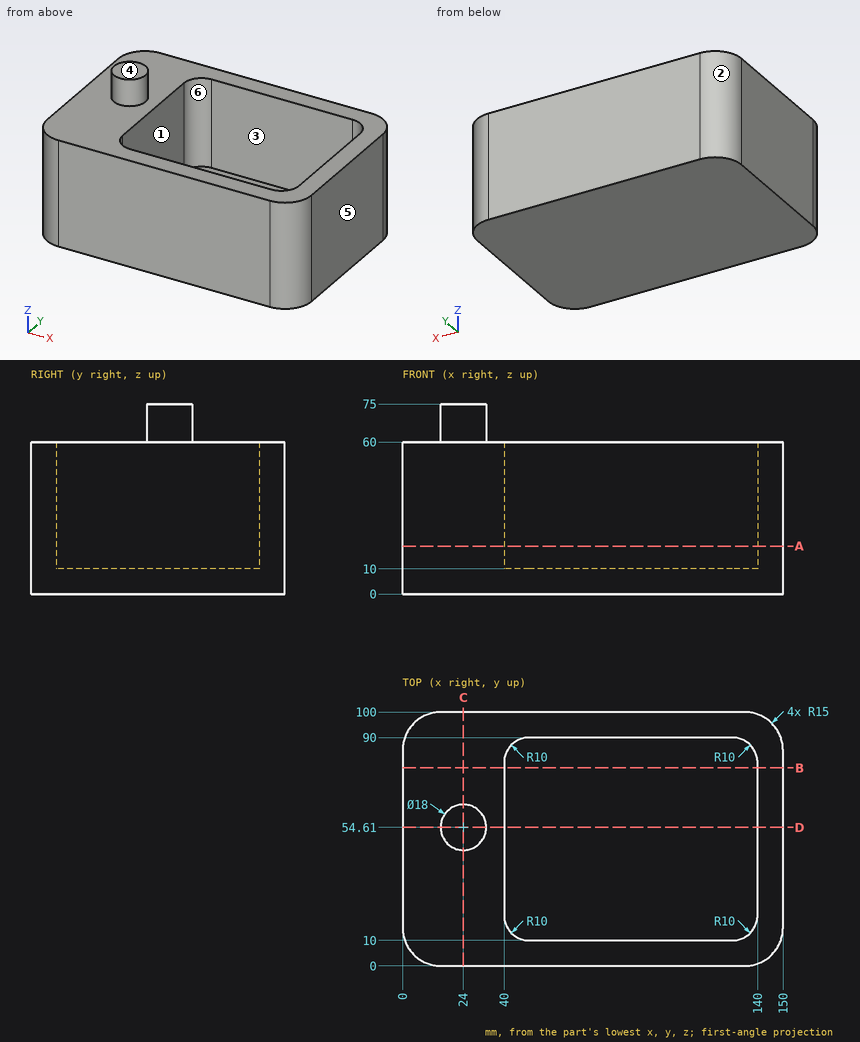
Geometry check sheet. Reference: drawing and pictorial views, mm from the part's lowest x, y, z. A direction names the side the tool comes from. Round coordinates to 2 decimals unless told otherwise and drop trailing zeros. Loops run counter-clockwise (first coordinate to the right, second up) from the corner with the lowest first, then second, coordinate; pieces in that order, holes last. Notation, with made-up numbers: (12, -10.5) - (64, -10.5) arc R19 ccw to (64, -1.5) - close; hole circle Ø1 at (47, 79.5). An arc over 180 degrees is marked (long way). Write item = value, one per line. Start each with the question number.
Q1. Release check for a two-part mould opening along Y. For the marked faces 1, 2, 3 and 4 record: pulls with the +Y half, pulls with the -Y half, needs draft (parallel to the pull), parting line crosses it, or undercut.
Q2. Depth check by flat-ended pin: P1, Ø4, axis at x = 62, y = 23.5, coming from the +Z side; P2, Ø3, axis at x = 17.5, y = 30.5, coming from the +Z side. Enter the tip coordinate at first touch or a pass-through.
Q3. Section check A-A (z = 19). Record the boundary of the cut face in (x, y).
Q4. Section check B-B (y = 78). Record the boundary of the cut face in (x, z), plus the area to 3 significant figures.
Q5. Section check C-C (x = 24). Record the boundary of the cut face in (y, z).
Q6. Access from +Z, -Z, +X, -X, +Y, -Y to the whole of each face (thin tool, end or side, straight path). Record for the marked faces 5 and 6.
Q7. Thickness scan on L1, parallel to X at y = 19.5, z = 50.5; L2, parallel to Y at x = 122.5, z = 38; L3, parallel to Y at x = 14, z = 21.5. Record the ranges inside material, lowest first.
Q8. Section check D-D (y = 54.61). Record the boundary of the cut face in (x, z).
Derived:
q1.face_1 = undercut
q1.face_2 = pulls with the +Y half
q1.face_3 = undercut
q1.face_4 = needs draft
q2.P1 = 10
q2.P2 = 60
q3.outline = (0, 15) arc R15 ccw to (15, 0) - (135, 0) arc R15 ccw to (150, 15) - (150, 85) arc R15 ccw to (135, 100) - (15, 100) arc R15 ccw to (0, 85) - close; hole (40, 20) arc R10 ccw to (50, 10) - (130, 10) arc R10 ccw to (140, 20) - (140, 80) arc R10 ccw to (130, 90) - (50, 90) arc R10 ccw to (40, 80) - close
q4.outline = (0, 0) - (150, 0) - (150, 60) - (140, 60) - (140, 10) - (40, 10) - (40, 60) - (0, 60) - close
q4.area = 4,000 mm^2
q5.outline = (0, 0) - (100, 0) - (100, 60) - (63.61, 60) - (63.61, 75) - (45.61, 75) - (45.61, 60) - (0, 60) - close
q6.face_5 = +Z, -Z, +X, +Y, -Y
q6.face_6 = +Z
q7.L1 = 0 to 40.01, 139.99 to 150
q7.L2 = 0 to 10, 90 to 100
q7.L3 = 0.03 to 99.97
q8.outline = (0, 0) - (150, 0) - (150, 60) - (140, 60) - (140, 10) - (40, 10) - (40, 60) - (33, 60) - (33, 75) - (15, 75) - (15, 60) - (0, 60) - close
